Part model, mm, in its own coordinate system. Round coordinates to 2 decimals unless told otherwise and drop trailing zeros. Write each loop counter-clockwise with the first axis right and the second up, starting at its lowest first coordinate (ties: lowest second). Pieces come first, ordered by that corner, then holes.
```python
from build123d import *

# Parameters (mm, degrees)
F2_DEPTH = 24.5
F3_ANGLE = 180


with BuildPart() as f2:
    # F1 (on Front) → F2 (new body)
    with BuildSketch(Plane.XZ):
        Polygon((0, 19), (0, 0), (-19, 0), (-19, -0.75), (-0.75, -0.75), (-0.75, -19), (0.75, -19), (0.75, -0.75), (19, -0.75), (19, 0.75), (0.75, 0.75), (0.75, 19), align=None)
        Polygon((-19, 0), (0, 0), (0, 19), (-0.75, 19), (-0.75, 0.75), (-19, 0.75), align=None)
    extrude(amount=F2_DEPTH)


with BuildPart() as f3:
    # F0 (on Front) → F3 (revolve)
    with BuildSketch(Plane.XZ):
        with BuildLine():
            Line((0, -20), (0, 0))
            Line((0, 0), (0, 20))
            ThreePointArc((0, 20), (-20, 0), (0, -20))
        make_face()
    revolve(axis=Axis((0, 0, 10), (0, 0, 1)), revolution_arc=F3_ANGLE)


with BuildPart() as f2_1:
    add(f2.part)

    # F4: cut F3
    add(f3.part, mode=Mode.SUBTRACT)


solid = f3.part
```
Q1. Cut at A-A on z = -16. Write the cut outline in (x, y), plus the area to 3 significant figures.
Values follow:
outline: (-12, 0) arc R12 ccw to (12, 0) - close
area: 226 mm2
Q2. Cut at B-B on y = -14.75. Write the cut outline in (x, z).
Values follow:
outline: circle Ø27.01 at (0, 0)
Q3. Cut at D-D on y = -17. Write the cut outline in (x, z), plus the area to 3 significant figures.
Values follow:
outline: circle Ø21.07 at (0, 0)
area: 349 mm2
Q4. Cut at C-C on x = -2.5. Write the cut outline in (y, z).
Values follow:
outline: (0, -19.84) - (0, 19.84) arc R19.84 ccw to start
Q5. Wall check: L1, parallel to Y at x = 9.5, z = 9.5; L2, parallel to Z at x = -10, y = -3.75; L3, parallel to Z at x = 8.5, y = -14. Give the ranges that are in metal, low to high.
Values follow:
L1: y = -14.82 to 0
L2: z = -16.91 to 16.91
L3: z = -11.48 to 11.48
Q6. Drop flat-ended pins along their axis: pin 1 (8 mm diameter, centred on y = -4, z = -9.5, fed in from -X); pin 2 (8 mm diameter, centred on y = -3.5, z = -15.5, fed in from +X); pin 3 (10 mm diameter, centred on x = 7.5, z = 4.5, fed in from -Y). Give the stop position or say it passes through.
Values follow:
pin 1: stops at x = -18.98
pin 2: stops at x = 16.08
pin 3: stops at y = -19.65
